Autodesk Inventor part; units mm, degrees
ref_plane "YZ Plane" through (0, 0, 0) normal (1, 0, 0) x (0, 1, 0)
ref_plane "XZ Plane" through (0, 0, 0) normal (0, 1, 0) x (-1, 0, 0)
ref_plane "XY Plane" through (0, 0, 0) normal (0, 0, 1) x (1, 0, 0)
sketch "Эскиз1" plane through (0, 0, 0) normal (0, 0, 1) x (1, 0, 0)
  line L0 (0, 0) -> (106.3, 0)
  line L1 (106.3, 0) -> (106.3, 62)
  line L2 (106.3, 62) -> (0, 62)
  line L3 (0, 62) -> (0, 0)
  dimension "d0" = 106.3
  dimension "d1" = 62
extrude "Выдавливание1" add sketch "Эскиз1" along normal blind 4
sketch "Эскиз2" plane through (0, 0, 4) normal (0, 0, 1) x (1, 0, 0)
  line L0 (106.3, 10) -> (106.3, 20)
  line L1 (110.3, 10) -> (106.3, 10)
  line L2 (110.3, 20) -> (110.3, 10)
  line L3 (110.3, 20) -> (106.3, 20)
  line L4 (106.3, 30) -> (106.3, 40)
  line L5 (110.3, 30) -> (106.3, 30)
  line L6 (110.3, 40) -> (110.3, 30)
  line L7 (110.3, 40) -> (106.3, 40)
  line L8 (106.3, 50) -> (106.3, 60)
  line L9 (110.3, 50) -> (106.3, 50)
  line L10 (110.3, 60) -> (110.3, 50)
  line L11 (110.3, 60) -> (106.3, 60)
  line L12 (-4, 10) -> (-4, 20)
  line L13 (0, 10) -> (-4, 10)
  line L14 (0, 20) -> (0, 10)
  line L15 (0, 20) -> (-4, 20)
  line L16 (-4, 30) -> (-4, 40)
  line L17 (0, 30) -> (-4, 30)
  line L18 (0, 40) -> (0, 30)
  line L19 (0, 40) -> (-4, 40)
  line L20 (-4, 50) -> (-4, 60)
  line L21 (0, 50) -> (-4, 50)
  line L22 (0, 60) -> (0, 50)
  line L23 (0, 60) -> (-4, 60)
  point P0 (0, 0)
extrude "Выдавливание2" add sketch "Эскиз2" against normal up to surface (4 mm away)
sketch "Эскиз3" plane through (-4, 50, 4) normal (-1, 0, 0) x (0, 0, 1)
  line L0 (-4, 10) -> (0, 10)
  line L1 (0, 10) -> (0, 16)
  line L2 (0, 16) -> (-10, 16.6879)
  line L3 (-10, 16.6879) -> (-10, 12.6879)
  line L4 (-10, 12.6879) -> (-20, 13.3759)
  line L5 (-20, 13.3759) -> (-20, 17.3759)
  line L6 (-20, 17.3759) -> (-30, 18.0638)
  line L7 (-30, 18.0638) -> (-30, 14.0638)
  line L8 (-30, 14.0638) -> (-40, 14.7517)
  line L9 (-40, 14.7517) -> (-40, 18.7517)
  line L10 (-40, 18.7517) -> (-50, 19.4397)
  line L11 (-50, 19.4397) -> (-50, 15.4397)
  line L12 (-50, 15.4397) -> (-60, 16.1276)
  line L13 (-60, 16.1276) -> (-60, 20.1276)
  line L14 (-60, 20.1276) -> (-70, 20.8155)
  line L15 (-70, 20.8155) -> (-70, 16.8155)
  line L16 (-70, 16.8155) -> (-80, 17.5035)
  line L17 (-80, 17.5035) -> (-80, 21.5035)
  line L18 (-80, 21.5035) -> (-90, 22.1914)
  line L19 (-90, 22.1914) -> (-90, 18.1914)
  line L20 (-90, 18.1914) -> (-100, 18.8794)
  line L21 (-100, 18.8794) -> (-100, 22.8794)
  line L22 (-100, 22.8794) -> (-110, 23.5673)
  line L23 (-110, 23.5673) -> (-110, 19.5673)
  line L24 (-110, 19.5673) -> (-120, 20.2552)
  line L25 (-120, 20.2552) -> (-120, 24.2552)
  line L26 (-120, 24.2552) -> (-130, 24.9432)
  line L27 (-130, 24.9432) -> (-130, 20.9432)
  line L28 (-130, 20.9432) -> (-140, 21.6311)
  line L29 (-140, 21.6311) -> (-140, 25.6311)
  line L30 (-140, 25.6311) -> (-145.3625, 26)
  line L31 (-145.3625, 26) -> (-145.3625, 16)
  line L32 (-145.3625, 16) -> (-208, -30)
  line L33 (-208, -50) -> (-208, -30)
  line L34 (-187, -50) -> (-208, -50)
  line L35 (-187, -54) -> (-187, -50)
  line L36 (-177, -54) -> (-187, -54)
  line L37 (-177, -50) -> (-177, -54)
  line L38 (-167, -50) -> (-177, -50)
  line L39 (-167, -54) -> (-167, -50)
  line L40 (-157, -54) -> (-167, -54)
  line L41 (-157, -50) -> (-157, -54)
  line L42 (-147, -50) -> (-157, -50)
  line L43 (-147, -54) -> (-147, -50)
  line L44 (-137, -54) -> (-147, -54)
  line L45 (-137, -50) -> (-137, -54)
  line L46 (-127, -50) -> (-137, -50)
  line L47 (-127, -54) -> (-127, -50)
  line L48 (-117, -54) -> (-127, -54)
  line L49 (-117, -50) -> (-117, -54)
  line L50 (-107, -50) -> (-117, -50)
  line L51 (-107, -54) -> (-107, -50)
  line L52 (-97, -54) -> (-107, -54)
  line L53 (-97, -50) -> (-97, -54)
  line L54 (-87, -50) -> (-97, -50)
  line L55 (-87, -54) -> (-87, -50)
  line L56 (-77, -54) -> (-87, -54)
  line L57 (-77, -50) -> (-77, -54)
  line L58 (-67, -50) -> (-77, -50)
  line L59 (-67, -54) -> (-67, -50)
  line L60 (-57, -54) -> (-67, -54)
  line L61 (-57, -50) -> (-57, -54)
  line L62 (-47, -50) -> (-57, -50)
  line L63 (-47, -54) -> (-47, -50)
  line L64 (-37, -54) -> (-47, -54)
  line L65 (-37, -50) -> (-37, -54)
  line L66 (-27, -50) -> (-37, -50)
  line L67 (-27, -54) -> (-27, -50)
  line L68 (-17, -54) -> (-27, -54)
  line L69 (-17, -50) -> (-17, -54)
  line L70 (-17, -50) -> (0, -50)
  line L71 (0, -50) -> (0, -40)
  line L72 (0, -40) -> (-4, -40)
  line L73 (-4, -40) -> (-4, -30)
  line L74 (-4, -30) -> (0, -30)
  line L75 (0, -30) -> (0, -20)
  line L76 (0, -20) -> (-4, -20)
  line L77 (-4, -20) -> (-4, -10)
  line L78 (-4, -10) -> (0, -10)
  line L79 (0, -10) -> (0, 0)
  line L80 (0, 0) -> (-4, 0)
  line L81 (-4, 0) -> (-4, 10)
  line L82 (-4, 12) -> (0, 12)
  line L83 (0, 12) -> (-10, 12.6879)
  line L84 (-4, 12) -> (-4, 13.5119)
  point P0 (-4, -50)
  point P1 (-4, 12.2752)
extrude "Выдавливание3" add sketch "Эскиз3" against normal up to surface (110.3 mm away) contours L82 L84 L83
sketch "Эскиз4" plane through (-4, 50, 4) normal (-1, 0, 0) x (0, 0, 1)
  line L0 (-4, 12) -> (0, 12)
  line L1 (0, 12) -> (-4, 12.2752)
  line L2 (-4, 12.2752) -> (-4, 12)
  point P0 (-4, -50)
extrude "Выдавливание4" cut sketch "Эскиз4" against normal up to surface (4 mm away)
properties part number "стульчак 4"
Design review of the part built by this model. Coordinates are the model's own, in mm. A direction names the side the tool comes from. Coordinates: 2 decimals unless noted, no trailing zeros. Loops run counter-clockwise (first coordinate to the right, second up) from the corner with the lowest first, then second, coordinate; pieces in that order, holes last. Notation, with made-up numbers: (19.5, 69) -> (57.5, 69) arc R29 ccw to (57.5, 91) -> close; hole circle Ø1 at (30, 30). An arc over 180 degrees is marked (long way). Use a Markdown table: item, result. Add a question column.
Item 1: The part is to be moulded in two halves that separate along Y. For faces 5 (the flat face through (-2, 10, 2)), 6 (the flat face through (110.3, 35, 2)), 7 (the flat face through (-2, 60, 2)), 8 (the flat face through (0, 45, 2)), say which applies: +Y half, -Y half, draft (parallel to the pull), parting line (faces both ways), or undercut.
Item 2: We need section A-A, the plane z = 0.65. Write out the cut boundary in (x, y).
Item 3: Machinability: for faces 1 (the flat face through (108, 10, 2)), 2 (the flat face through (106.3, 61, 2)), 3 (the flat face through (-2, 50, 2)), 4 (the flat face through (0, 5, 2)), which of the approach directions +Z, -Z, +X, -X, +Y, -Y give a long, thin tool a straight path to every point of the face, cutting with its end or side? Answer none if there is none.
Item 4: We need section B-B, the plane y = 42. Write out the cut boundary in (x, z), and give its area (3 significant figures).
Item 5: Clearance check with flat-ended pins moving along their axes: P1, Ø2, axis at x = -2, z = 1.5, coming from the +Y side; P2, Ø2, axis at y = 5.5, z = 2, coming from the -X side; P3, Ø2, axis at y = 25, z = 2.5, coming from the +X side. State where each tip first meets the part, or that it passes through.
Item 6: Wall thickness on L1, parallel to X at y = 4, z = 2.55; L2, parallel to Y at x = 86, z = 0.2; L3, parallel to Y at x = 4, z = 2.25: over which ranges is each line inside the solid? List them lowest first. Write a range as from..to.
Numbers:
| question | item | result |
|---|---|---|
| 1 | face 5 | -Y half |
| 1 | face 6 | draft |
| 1 | face 7 | +Y half |
| 1 | face 8 | undercut |
| 2 | outline | (-4, 10) -> (0, 10) -> (0, 0) -> (106.3, 0) -> (106.3, 10) -> (110.3, 10) -> (110.3, 20) -> (106.3, 20) -> (106.3, 30) -> (110.3, 30) -> (110.3, 40) -> (106.3, 40) -> (106.3, 50) -> (110.3, 50) -> (110.3, 60) -> (106.3, 60) -> (106.3, 62.23) -> (0, 62.23) -> (0, 60) -> (-4, 60) -> (-4, 50) -> (0, 50) -> (0, 40) -> (-4, 40) -> (-4, 30) -> (0, 30) -> (0, 20) -> (-4, 20) -> close |
| 3 | face 1 | +Z, -Z, +X, -Y |
| 3 | face 2 | +Z, -Z, +X, +Y |
| 3 | face 3 | +Z, -Z, -X |
| 3 | face 4 | +Z, -Z, -X, -Y |
| 4 | outline | (0, 0) -> (106.3, 0) -> (106.3, 4) -> (0, 4) -> close |
| 4 | area | 425 mm^2 |
| 5 | P1 | stops at y = 60 |
| 5 | P2 | stops at x = 0 |
| 5 | P3 | stops at x = 106.3 |
| 6 | L1 | x = 0..106.3 |
| 6 | L2 | y = 0..62.26 |
| 6 | L3 | y = 0..62.12 |
